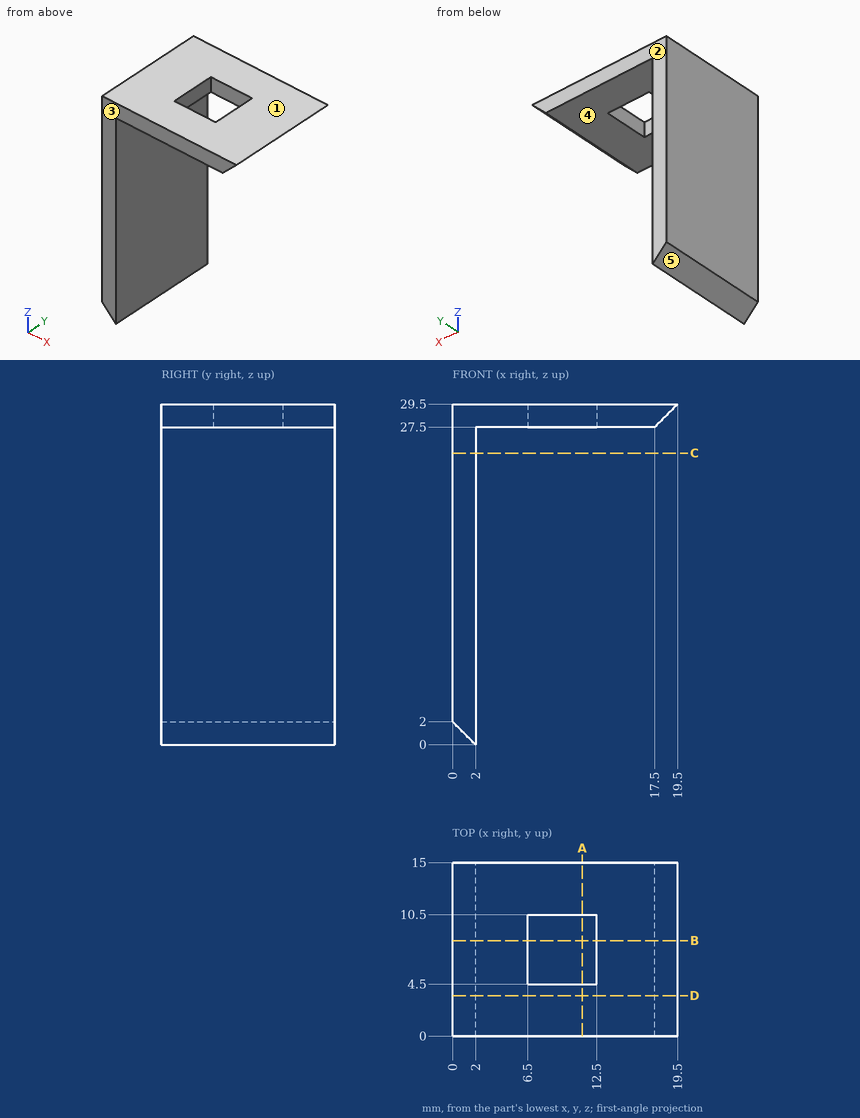
Here's the drawing with two shaded views (mm, measured from the low corner). I have some questions. A direction names the side the tool comes from. Give positions to 0.01 mm unless a question says otherwise; leave off trailing zeros. Loops run counter-clockwise (first coordinate to the right, second up) from the corner with the lowest first, then second, coordinate; pieces in that order, holes last. Notation, with made-up numbers: (-17.75, 29) -> (4.25, 29) arc R23 cw to (4.25, 65) -> close; hole circle Ø9 at (-40, 31.5). An arc over 180 degrees is marked (long way). Answer as a JSON object with one key per item and string values. Group by question number.
Item 1: Imagine slicing it at D-D on y = 3.5. Write out the boundary of the cut face in (x, z), then the cut area to 3 significant figures.
Item 2: Imagine slicing it at A-A on x = 11.25. Write out the boundary of the cut face in (y, z), then the cut area to 3 significant figures.
Item 3: Imagine slicing it at C-C on z = 25.25. Write out the boundary of the cut face in (x, y).
Item 4: Will these pins go through, and if not, where does the flat tip stop? pin 1 (3 mm diameter, centred on x = 12.5, y = 7, fed in from -Z); pin 2 (7.5 mm diameter, centred on y = 4, z = 13.5, fed in from +X); pin 3 (1.5 mm diameter, centred on x = 3.5, z = 15.5, fed in from -Y).
Item 5: Thinking about a two-plate mould opening in Y: for the marked faces 1, 2 and 3, which applies, pulls with the +Y half, pulls with the -Y half, needs draft (parallel to the pull), parting line crosses it, or undercut?
Item 6: I need wall thicknesses on L1, parallel to X at y = 3.75, z = 19.75; L2, parallel to Z at x = 5.75, y = 13.25; L3, parallel to Z at x = 1.25, y = 11. Which ranges of each line are inside material? Lowest first, please.
Item 7: Imagine slicing it at B-B on y = 8.25. Write out the boundary of the cut face in (x, z).
Item 8: On a 3-axis mill with a long thin cutter (end or side, diameter ignored), from which of +Z, -Z, +X, -X, +Y, -Y can I reach the whole of each face in a straight line? I mean the marked faces 4 and 5. Say none if no direction works.
Answer list:
{
 "1": {"outline": "(0, 2) -> (2, 0) -> (2, 27.5) -> (17.5, 27.5) -> (19.5, 29.5) -> (0, 29.5) -> close", "area": "90.0 mm2"},
 "2": {"outline": "(0, 27.5) -> (4.5, 27.5) -> (4.5, 29.5) -> (0, 29.5) -> close; (10.5, 27.5) -> (15, 27.5) -> (15, 29.5) -> (10.5, 29.5) -> close", "area": "18.0 mm2"},
 "3": {"outline": "(0, 0) -> (2, 0) -> (2, 15) -> (0, 15) -> close"},
 "4": {"pin 1": "stops at z = 27.5", "pin 2": "stops at x = 2", "pin 3": "passes through"},
 "5": {"face 1": "needs draft", "face 2": "pulls with the +Y half", "face 3": "pulls with the -Y half"},
 "6": {"L1": "x = 0 to 2", "L2": "z = 27.5 to 29.5", "L3": "z = 0.75 to 29.5"},
 "7": {"outline": "(0, 2) -> (2, 0) -> (2, 27.5) -> (6.5, 27.5) -> (6.5, 29.5) -> (0, 29.5) -> close; (12.5, 27.5) -> (17.5, 27.5) -> (19.5, 29.5) -> (12.5, 29.5) -> close"},
 "8": {"face 4": "-Z, +X, +Y, -Y", "face 5": "-Z, -X, +Y, -Y"}
}
